from build123d import *


with BuildPart() as f1:
    # F0 (on Front) → F1 (revolve)
    with BuildSketch(Plane.XZ):
        with BuildLine():
            Line((-127, 0), (0, 0))
            Line((0, 0), (0, 419.1))
            ThreePointArc((0, 419.1), (-17.960512, 411.660512), (-25.4, 393.7))
            Line((-25.4, 393.7), (-25.4, 63.5))
            ThreePointArc((-25.4, 63.5), (-32.839488, 45.539488), (-50.8, 38.1))
            Line((-50.8, 38.1), (-152.4, 38.1))
            ThreePointArc((-152.4, 38.1), (-170.360512, 30.660512), (-177.8, 12.7))
            Line((-177.8, 12.7), (-177.8, -38.1))
            Line((-177.8, -38.1), (-127, -38.1))
            Line((-127, -38.1), (-127, 0))
        make_face()
    revolve(axis=Axis((0, 0, 209.55), (0, 0, -1)))


solid = f1.part
Build history of the part. All positions in model axes, mm. A direction names the side the tool comes from. Give positions to 0.01 mm unless a question says otherwise; leave off trailing zeros. Loops run counter-clockwise (first coordinate to the right, second up) from the corner with the lowest first, then second, coordinate; pieces in that order, holes last. Notation, with made-up numbers: (72.25, 57.25) - (114.25, 57.25) arc R14 ccw to (114.25, 80.25) - close; hole circle Ø6 at (57, 28). An arc over 180 degrees is marked (long way). Write item = value, one per line. Start each with the question number.
1) Probe probe 1 along Y at (x, z) = (0, -13.5); probe 2 along Z at (x, y) = (107.5, 17); probe 3 along X at (y, z) = (23.5, 184). List the from-to ranges inside material, lowest first. Write a range as from..to.
2) Drop flat-ended pins along their axis: pin 1 Ø3 at (x, y) = (46.5, -80) entering from -Z; pin 2 Ø6 at (y, z) = (19, 105) entering from +X; pin 3 Ø10 at (x, y) = (-37.5, -124) entering from +Z. Give the stop position or say it passes through.
3) Band-saw the part on A-A on z = 383. Give the cut face in (x, y).
4) Pull direction X, two halves, no side cores. Call faces 1 (the flat face through (2, 2, 0)), 2 (the flat face through (121, 42, -38.1)), 3 (the cylindrical face through (-169.59, 53.41, -13.06)): +X half, -X half, draft (parallel to the pull), parting line (faces both ways), or undercut.
5) Band-saw the part on B-B on z = 45. Give the cut face in (x, y), plus the area to 3 significant figures.
6) Tool access for faces 4 (the cylindrical face through (5.506, -24.796, 226.289)), 5 (the cylindrical face through (27.53, -123.98, -18.78)): list every direction of +Z, -Z, +X, -X, +Y, -Y with a clear straight run to the whole face (end or side of a thin tool).
Final values:
q1.probe_1 = -177.8..-127, 127..177.8
q1.probe_2 = 0..38.1
q1.probe_3 = -9.64..9.64
q2.pin_1 = 0
q2.pin_2 = 19.73
q2.pin_3 = 38.1
q3.outline = circle Ø50.8 at (0, 0)
q4.face_1 = undercut
q4.face_2 = draft
q4.face_3 = parting line
q5.outline = circle Ø66.79 at (0, 0)
q5.area = 3,500 mm²
q6.face_4 = +Z
q6.face_5 = -Z
